Work out the finished part from the listing and answer in its coordinate system (mm). Coordinates: 2 decimals unless noted, no trailing zeros. Order: outer loops, then holes, each group sorted by start corner. A loop starts at its lowest first (then second) coordinate and runs counter-clockwise, first axis right, second up. Notation, with made-up numbers: (2, -32.75) -> (53, -32.75) arc R20 cw to (53, -16.75) -> close; hole circle Ø10 at (-38, 24.25). An arc over 180 degrees is marked (long way). Use one line per item in the form item = value.
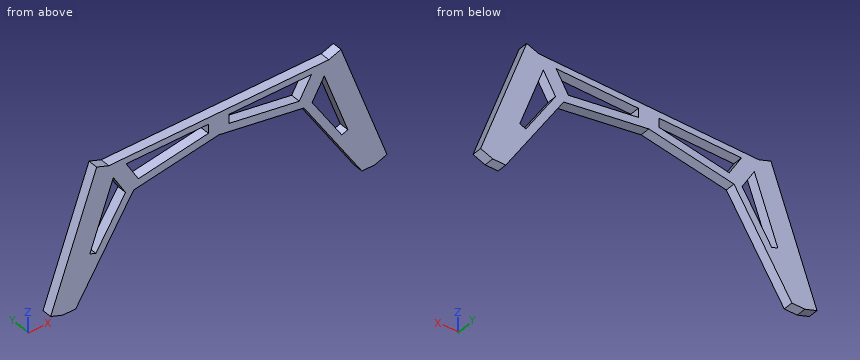
from build123d import *

# Parameters (mm, degrees)
F2_DEPTH = 19.05


# Not quite as in the source:
# - a variable given as a bare number and used for a length is read in inches; the dataset says mm whatever the document's units were


with BuildPart() as f2:
    # F1 (on Front) → F2 (new body)
    with BuildSketch(Plane.XZ):
        Polygon((215.9, 0), (0, 0), (-215.9, 0), (-306.2480410609, -248.2292027068), (-280.8480410609, -248.2292027068), (-167.1250061285, -70.7126014387), (0, -43.18), (167.1250061285, -70.7126014387), (280.8480410609, -248.2292027068), (306.2480410609, -248.2292027068), align=None)
        Polygon((-253.2563468183, -154.4156124752), (-207.0382383225, -27.4324030132), (-183.0905760207, -67.8622134293), (-241.3222505343, -158.7592682954), align=None, mode=Mode.SUBTRACT)
        Polygon((-181.84793878, -12.7), (-20.4141870137, -12.7), (-20.4141870137, -30.48), (-157.9002764782, -53.1298104161), align=None, mode=Mode.SUBTRACT)
        Polygon((183.0905760207, -67.8622134293), (207.0382383225, -27.4324030132), (253.2563468183, -154.4156124752), (241.3222505343, -158.7592682954), align=None, mode=Mode.SUBTRACT)
        Polygon((157.9002764782, -53.1298104161), (20.4141870137, -30.48), (20.4141870137, -12.7), (181.84793878, -12.7), align=None, mode=Mode.SUBTRACT)
        Polygon((-306.2480410609, -248.2292027068), (-215.9, 0), (-239.768192568, 8.6873116405), (-330.1162336289, -239.5418910663), align=None)
        Polygon((239.768192568, 8.6873116405), (215.9, 0), (306.2480410609, -248.2292027068), (330.1162336289, -239.5418910663), align=None)
    extrude(amount=F2_DEPTH)


solid = f2.part
(1) Each of these flat-tipped pins is pushed along its axis until it touches: P1, Ø9, axis at y = -12, z = -23, coming from the +X side; P2, Ø4, axis at x = -64, y = -17, coming from the -Z side; P3, Ø4, axis at y = -3, z = -138.5, coming from the +X side. Where does it stop, or does it pass through?
Data:
P1 = 252.94
P2 = -54.05
P3 = 294.07
(2) Straight lines are drawn through the part: line 1 along X through (y, z) = (-6.25, -120); line 2 along X through (y, z) = (-9, -147); line 3 along X through (y, z) = (-8.75, -19.5). For each, find the intervals that lie inside material, in ascending order.
Data:
line_1 = -286.61 to -240.73, -216.49 to -198.7, 198.7 to 216.49, 240.73 to 286.61
line_2 = -296.43 to -250.56, -233.79 to -216, 216 to 233.79, 250.56 to 296.43
line_3 = -250.03 to -177.82, -20.41 to 20.41, 177.82 to 250.03
(3) Section A-A on x = 105.5 is taken. Write down the section's boundary in (y, z), plus the area to 3 significant figures.
Data:
outline = (-19.05, -60.56) -> (0, -60.56) -> (0, -44.5) -> (-19.05, -44.5) -> close; (-19.05, -12.7) -> (0, -12.7) -> (0, 0) -> (-19.05, 0) -> close
area = 548 mm²
(4) Section B-B on y = -5.5 is taken. Count the separate pieces of the cut face and the enclosed holes in it, plus the area to 3 significant figures.
Data:
separate_pieces = 1
enclosed_holes = 4
area = 43,700 mm²
(5) Section C-C on z = -102.5 is taken. Write down the section's boundary in (x, y), plus the area to 3 significant figures.
Data:
outline = (-280.24, -19.05) -> (-234.36, -19.05) -> (-234.36, 0) -> (-280.24, 0) -> close; (-205.28, -19.05) -> (-187.49, -19.05) -> (-187.49, 0) -> (-205.28, 0) -> close; (187.49, -19.05) -> (205.28, -19.05) -> (205.28, 0) -> (187.49, 0) -> close; (234.36, -19.05) -> (280.24, -19.05) -> (280.24, 0) -> (234.36, 0) -> close
area = 2,430 mm²
